Input: part model. Units: mm. Frame: model coordinates. A direction names the side the tool comes from. Give positions to 0.01 mm unless a question says otherwise; leave off trailing zeros. Loops run counter-clockwise (first coordinate to the right, second up) from the corner with the lowest first, then second, coordinate; pieces in that order, holes last. Notation, with made-up numbers: (22, 29.25) - (43, 29.25) arc R23 ccw to (43, 43.25) - close; hole circle Ø6 at (51.25, 37). An arc over 180 degrees is marked (long way). One line per item, written item: value.
Autodesk Inventor part; units mm, degrees
ref_plane "YZ Plane" through (0, 0, 0) normal (1, 0, 0) x (0, 1, 0)
ref_plane "XZ Plane" through (0, 0, 0) normal (0, 1, 0) x (-1, 0, 0)
ref_plane "XY Plane" through (0, 0, 0) normal (0, 0, 1) x (1, 0, 0)
sketch "Sketch1" plane through (0, 0, 0) normal (0, 0, 1) x (1, 0, 0)
  line L0 (-28.9877, 0) -> (173.9264, 0)
  line L1 (-29.4372, -7.8877) -> (176.6233, 47.3261)
  line L2 (101.2142, 39.5436) -> (111.8098, 0)
  line L3 (111.8098, 0) -> (144.9387, 0)
  line L4 (144.9387, 0) -> (132.1238, 47.8258)
  line L5 (132.1238, 47.8258) -> (123.4305, 45.4964)
  line L6 (123.4305, 45.4964) -> (132.4891, 11.689)
  line L7 (109.9075, 41.8729) -> (118.9662, 8.0655)
  line L8 (118.9662, 8.0655) -> (132.4891, 11.689)
  line L9 (109.9075, 41.8729) -> (101.2142, 39.5436)
  point P0 (0, 0)
  point P1 (132.0574, 26.729)
  point P2 (96.5926, 25.8819)
  dimension "d0" = 12
  dimension "d1" = 9
  dimension "d2" = 14
  dimension "d3" = 9
  dimension "d4" = 35
  dimension "d5" = 117
extrude "Extrusion1" add sketch "Sketch1" along normal mid plane 50 contours L2 L1 L7 L8 L6 L4 L0 | L2 L9 L7 L1 | L1 L6 L5 L4
sketch "Sketch3" plane through (111.8098, 0, -25) normal (-0.9659, -0.2588, 0) x (0, 0, 1)
  line L0 (25, 64.8401) -> (25, -46.4712)
  line L1 (50, 40.9385) -> (0, 40.9385)
  line L2 (50, -8.5744) -> (0, -8.5744)
  line L3 (50, 40.9385) -> (0, 40.9385)
  line L4 (1.57, -23.5744) -> (48.43, -23.5744)
  line L5 (1.57, -23.5744) -> (13.2622, 31.4335)
  line L6 (48.43, -23.5744) -> (36.7378, 31.4335)
  arc A0 (36.7378, 31.4335) -> (13.2622, 31.4335) centre (25, 28.9385) ccw
  dimension "d8" = 12
  dimension "d9" = 78
  dimension "d10" = 78
  dimension "d12" = 15
extrude "Extrusion2" cut sketch "Sketch3" against normal through all keep common part
sketch "Sketch4" plane through (0, 0, 0) normal (0, 0, 1) x (1, 0, 0)
  point P0 (0, 0)
sketch "Sketch5" plane through (0, 0, 0) normal (0, 0, 1) x (1, 0, 0)
  point P0 (0, 0)
sketch "Sketch6" plane through (0, 0, 0) normal (0, 0, 1) x (1, 0, 0)
  line L0 (-28.9877, 0) -> (173.9264, 0)
  point P0 (0, 0)
sketch "Sketch7" plane through (0, 0, 0) normal (0, 0, 1) x (1, 0, 0)
  line L0 (-28.9877, 0) -> (173.9264, 0)
  line L1 (-29.4372, -7.8877) -> (176.6233, 47.3261)
  line L2 (132.9832, 25.3) -> (139.7623, 0)
  line L3 (139.7623, 0) -> (195.6672, 0)
  line L4 (195.6672, 0) -> (182.56, 48.9168)
  line L5 (182.56, 48.9168) -> (153.5822, 41.1522)
  line L6 (153.5822, 41.1522) -> (156.1654, 31.5117)
  line L7 (156.1654, 31.5117) -> (132.9832, 25.3)
  line L8 (134.5839, 38.6446) -> (144.9387, 0)
  line L9 (132.1238, 47.8258) -> (134.5839, 38.6446)
  point P0 (0, 0)
  dimension "d15" = 5
  dimension "d16" = 49
  dimension "d17" = 30
  dimension "d18" = 25.3
extrude "Extrusion3" add sketch "Sketch7" along normal mid plane 61 contours L2 L7 L8 L0 | L8 L7 L6 L1 L5 L4 L3 L0
sketch "Sketch8" plane through (153.5822, 41.1522, 30.5) normal (-0.2588, 0.9659, 0) x (0.9659, 0.2588, 0)
  line L0 (-19, 56) -> (35, 56)
  line L1 (35, 56) -> (35, 5)
  line L2 (35, 5) -> (-19, 5)
  line L3 (-19, 5) -> (-19, 56)
  line L4 (0, 61) -> (30, 61)
  line L5 (30, 61) -> (30, 0)
  line L6 (30, 0) -> (0, 0)
  line L7 (0, 61) -> (0, 0)
  line L8 (-24, 0) -> (-24, 16.1105)
  line L9 (-24, 61) -> (0, 61)
  point P0 (-159, 30.5)
  dimension "d23" = 5
  dimension "d25" = 5
  dimension "d26" = 5
  dimension "d28" = 5
extrude "Extrusion4" cut sketch "Sketch8" against normal through all contours L0 L7 L2 L3 | L0 L5 L2 L7 | L0 L1 L2 L5
sketch "Sketch9" plane through (0, 0, 0) normal (0, 0, 1) x (1, 0, 0)
  line L0 (153.5822, 41.1522) -> (182.56, 48.9168)
  line L1 (182.56, 48.9168) -> (195.6672, 0)
  line L2 (-39.5137, -10.5877) -> (237.0823, 63.526)
  line L3 (195.6672, 0) -> (182.56, 48.9168)
  line L4 (182.56, 48.9168) -> (153.5822, 41.1522)
  circle A0 centre (168.0711, 45.0345) radius 15
  point P0 (0, 0)
  dimension "d81" = 30
extrude "Extrusion5" add sketch "Sketch9" along normal mid plane 71
sketch "Sketch11" plane through (0, 0, 0) normal (0, 0, 1) x (1, 0, 0)
  circle A0 centre (168.0711, 45.0345) radius 19.5
  circle A1 centre (168.0711, 45.0345) radius 15
  point P0 (0, 0)
  dimension "d36" = 39
extrude "Extrusion6" cut sketch "Sketch11" along normal mid plane 41 contours A0 | A1
sketch "Sketch12" plane through (0, 0, 0) normal (0, 1, 0) x (-1, 0, 0)
  line L0 (-234.8006, 0) -> (39.1334, 0)
  line L1 (-195.6672, -30.5) -> (-195.6672, 30.5)
  line L2 (-195.6672, 30.5) -> (-91.6172, 42.9434)
  line L3 (-82.6672, 35) -> (-82.6672, -35)
  line L4 (-91.6172, -42.9434) -> (-195.6672, -30.5)
  arc A0 (-91.6172, -42.9434) -> (-82.6672, -35) centre (-90.6672, -35) ccw
  arc A1 (-82.6672, 35) -> (-91.6172, 42.9434) centre (-90.6672, 35) ccw
  point P0 (0, 0)
  dimension "d39" = 8
  dimension "d40" = 8
  dimension "d41" = 113
  dimension "d42" = 70
  dimension "d43" = 35
extrude "Extrusion7" add sketch "Sketch12" against normal blind 6
sketch "Sketch14" plane through (168.0711, 45.0345, -20.5) normal (0, 0, 1) x (1, 0, 0)
  circle A0 centre (0, 0) radius 15
  point P0 (-168.0711, -45.0345)
hole "Hole1" at (168.0711, 45.0345, -20.5) direction (0, 0, -1) diameter 15 end through all
sketch "Sketch15" plane through (168.0711, 45.0345, 35.5) normal (0, 0, 1) x (1, 0, 0)
  circle A0 centre (0, 0) radius 15
  point P0 (-168.0711, -45.0345)
hole "Hole2" at (168.0711, 45.0345, 35.5) direction (0, 0, -1) diameter 15 end through all
sketch "Sketch16" plane through (0, 0, 0) normal (0, 1, 0) x (1, 0, 0)
  arc A0 (91.6172, 42.9434) -> (82.6672, 35) centre (90.6672, 35) ccw
  point P0 (0, 0)
hole "Hole3" at (90.6672, 0, -35) direction (0, -1, 0) diameter 8 end through all
sketch "Sketch17" plane through (0, 0, 0) normal (0, 1, 0) x (1, 0, 0)
  arc A0 (82.6672, -35) -> (91.6172, -42.9434) centre (90.6672, -35) ccw
  point P0 (0, 0)
hole "Hole4" at (90.6672, 0, 35) direction (0, -1, 0) diameter 8 end through all
sketch "Sketch18" plane through (104.32, 27.9525, 0) normal (-0.9659, -0.2588, 0) x (0, 0, 1)
  arc A0 (11.7378, 2.4949) -> (-11.7378, 2.4949) centre (0, 0) ccw
  point P0 (0, 0)
hole "Hole5" at (104.32, 27.9525, 0) direction (0.9659, 0.2588, 0) diameter 9 end through all
equation "\"d81\" = d17"
equation "\"d36\" = 1.3 * d17"
equation "\"d43\" = 0.5 * d42"
properties part number "Reper" material "Steel, Carbon"
Item 1: Section D-D, the plane x = 93. Output: boundary loops of the cut face in (y, z), and give its area (3 significant figures).
Verdict:
outline: (-6, -42.78) - (0, -42.78) - (0, -38.25) - (-6, -38.25) - close; (-6, -31.75) - (0, -31.75) - (0, 31.75) - (-6, 31.75) - close; (-6, 38.25) - (0, 38.25) - (0, 42.78) - (-6, 42.78) - close
area: 435 mm^2
Item 2: Pin query (flat end, axial travel): P1, Ø19.5, axis at x = 168.07, y = 45.03, coming from the +Z side; P2, Ø9, axis at x = 173, y = 45, coming from the -Z side; P3, Ø4, axis at y = 29, z = 11.5, coming from the -X side. Return the tip coordinate at first contact, or that it passes through.
Verdict:
P1: stops at z = 35.5
P2: stops at z = -35.5
P3: stops at x = 103.5
Item 3: Draft query along Y for faces 1 (the face through (125.63, 9.85, -0.24)), 2 (the face through (144.371, -2.958, 36.635)), 3 (the face through (128.429, 43.986, 7.648)). Return one class per face: pulls with the +Y half, pulls with the -Y half, needs draft (parallel to the pull), parting line crosses it, or undercut.
Verdict:
face 1: undercut
face 2: needs draft
face 3: pulls with the +Y half
Item 4: Section B-B, the plane y = 14. Output: boundary loops of the cut face in (x, z), and give its area (3 significant figures).
Verdict:
outline: (108.06, -15.34) - (117.38, -15.85) - (117.38, 15.85) - (108.06, 15.34) - close; (131.87, -16.65) - (136.01, -16.88) - (136.01, -30.5) - (191.92, -30.5) - (191.92, -25.5) - (141.19, -25.5) - (141.19, 25.5) - (191.92, 25.5) - (191.92, 30.5) - (136.01, 30.5) - (136.01, 16.88) - (131.87, 16.65) - close
area: 1,250 mm^2
Item 5: Section A-A, the plane z = -33. Output: boundary loops of the cut face in (x, y), and give its area (3 significant figures).
Verdict:
outline: (82.67, -6) - (87.2, -6) - (87.2, 0) - (82.67, 0) - close; (94.13, -6) - (174.76, -6) - (174.76, 0) - (94.13, 0) - close; circle Ø30 at (168.07, 45.03); hole circle Ø15 at (168.07, 45.03)
area: 1,040 mm^2
Item 6: Access query for faces 4 (the face through (161, 42, -20.5)), 5 (the face through (117.118, 13.668, -15.905)), 6 (the face through (140.016, 18.371, 0.357)), 7 (the face through (166.118, 59.907, 28.105)), 8 (the face through (94.57, -3.04, 34.13)). Directions: +Z, -Z, +X, -X, +Y, -Y. A direction counts if a zero-diameter tool reaches every point of the face in a straight line with its end or side. Return the directions, or none.
Verdict:
face 4: +X, -X, +Y
face 5: -Z, -X
face 6: +X, +Y
face 7: none
face 8: +Y, -Y
Item 7: Material intervals for L1, parallel to Z at x = 158.5, y = 40.5; L2, parallel to Z at x = 159, y = 13; L3, parallel to Y at x = 146, z = -16, sorted ascending.
Verdict:
L1: z = -35.5 to -20.5, 20.5 to 35.5
L2: z = -30.5 to -25.5, 25.5 to 30.5
L3: y = -6 to 0
Item 8: Section C-C, the plane z = -22. Count the separate pieces of the cut face and the enclosed holes in it, and give its area (3 significant figures).
Verdict:
separate pieces: 2
enclosed holes: 1
area: 1,340 mm^2
